```python
from build123d import *

# Parameters (mm, degrees)
F0_R     = 6
F0_R_2   = 2
F1_DEPTH = 40
F0_R_3   = 12
F2_DEPTH = 4
F3_SIZE  = 1.99999


# Not quite as in the source:
# - a fillet or chamfer is up to 0.001 mm smaller than in the source, because OpenCascade refuses the exact size


with BuildPart() as f1:
    # F0 (on Top) → F1 (new body)
    with BuildSketch(Plane.XY):
        Circle(F0_R)
        Circle(F0_R_2, mode=Mode.SUBTRACT)
    extrude(amount=F1_DEPTH)

    # F0 (on Top) → F2 (join)
    with BuildSketch(Plane.XY):
        Circle(F0_R_3)
        Circle(F0_R, mode=Mode.SUBTRACT)
    extrude(amount=F2_DEPTH)

    # F3 (size 2 in the source; OpenCascade refuses exactly that, so slightly less here)
    f3_edges = [f1.edges().sort_by_distance(p)[0] for p in [
        (-6, 0, 40),
        (-2, 0, 40),
        (-2, 0, 0),
    ]]
    chamfer(f3_edges, length=F3_SIZE)


solid = f1.part
```
Geometry check sheet. Reference: the model listing, model coordinates, mm. Coordinates: 2 decimals unless noted, no trailing zeros. Write each loop counter-clockwise with the first axis right and the second up, starting at its lowest first coordinate (ties: lowest second). Pieces come first, ordered by that corner, then holes. Notation, with made-up numbers: M 5.5,32 L 62.5,32 A25 ccw 62.5,64 Z; hole C -13.5,30.5 d2. An arc over 180 degrees is marked long. Use one line per item in the form item = value. Start each with the question number.
1) Release check for a two-part mould opening along X. For faces 1 (the conical face through (-0.28, 2.11, 38.13)), 2 (the flat face through (-3, 3, 0)), 3 (the cylindrical face through (-11.99, 0.53, 1.97)), 4 (the cylindrical face through (0, -2, 20)) record: pulls with the +X half, pulls with the -X half, needs draft (parallel to the pull), parting line crosses it, or undercut.
2) Section check D-D on z = 25. Enter the section's corners in (x, y), and give its area (3 significant figures).
3) Section check C-C on z = 3.5. Enter the section's corners in (x, y), and give its area (3 significant figures).
4) Thickness scan on probe 1 along Y at (x, z) = (0, 29); probe 2 along Z at (x, y) = (-3, 11.25); probe 3 along X at (y, z) = (0.75, 34). Record the ranges inside material, lowest first. Write a range as from..to.
5) Go/stop test with flat-tipped pins: pin 1 Ø10 at (x, y) = (0, 2) entering from -Z; pin 2 Ø4.5 at (x, y) = (0, 0) entering from -Z; pin 3 Ø2 at (x, z) = (-8.5, 27.5) entering from +Y; pin 4 Ø5 at (x, z) = (-8, 34.5) entering from +Y. Record where each tip stops, or that it passes through.
Responses:
q1.face_1 = undercut
q1.face_2 = needs draft
q1.face_3 = parting line crosses it
q1.face_4 = undercut
q2.outline = C 0,0 d12; hole C 0,0 d4
q2.area = 101 mm2
q3.outline = C 0,0 d24; hole C 0,0 d4
q3.area = 440 mm2
q4.probe_1 = -6..-2, 2..6
q4.probe_2 = 0..4
q4.probe_3 = -5.95..-1.85, 1.85..5.95
q5.pin_1 = 0
q5.pin_2 = 1.75
q5.pin_3 = through
q5.pin_4 = 2.4
